Model file for the job. Use its own axes, mm. A direction names the side the tool comes from. Coordinates: 2 decimals unless noted, no trailing zeros. Order: outer loops, then holes, each group sorted by start corner. A loop starts at its lowest first (then second) coordinate and runs counter-clockwise, first axis right, second up. Notation, with made-up numbers: (75, 49) - (89, 49) arc R29 cw to (89, 77) - close; hole circle Ø8 at (66.5, 52.25). An arc over 180 degrees is marked (long way). Put each result on its own line as item: value. Start each with the question number.
```python
from build123d import *

# Parameters (mm, degrees)
SKETCH1_R           = 9.4615
BOSS_EXTRUDE1_DEPTH = 13.97
SKETCH2_R           = 1.905
CUT_EXTRUDE1_DEPTH  = 20.344272137
BOSS_EXTRUDE2_START = 15.24
SKETCH4_R           = 1.905
BOSS_EXTRUDE2_DEPTH = 15.24
FILLET1_R           = 25.4
SKETCH5_R           = 2.286
CUT_EXTRUDE2_DEPTH  = 33.12886653
SKETCH6_R           = 19.05
SKETCH6_R_2         = 9.4615
BOSS_EXTRUDE3_DEPTH = 2.54
SKETCH7_W           = 2.54
SKETCH7_H           = 7.62
CUT_EXTRUDE3_DEPTH  = 40.736999132
CIRPATTERN1_COUNT   = 2


with BuildPart() as part:
    # Sketch1 → Boss-Extrude1 (new body)
    with BuildSketch(Plane(origin=(0, 0, 0), x_dir=(1, 0, 0), z_dir=(0, 1, 0))):
        with Locations(Location((0, 0, 0), (0, 0, 270))):
            Circle(SKETCH1_R)
    extrude(amount=BOSS_EXTRUDE1_DEPTH)

    # Sketch2 → Cut-Extrude1 (cut, through all)
    with BuildSketch(Plane(origin=(0, 13.97, 0), x_dir=(1, 0, 0), z_dir=(0, 1, 0))):
        with Locations(Location((-4.064, 0, 0), (0, 0, 270))):
            Circle(SKETCH2_R)
        with Locations(Location((4.064, 0, 0), (0, 0, 270))):
            Circle(SKETCH2_R)
    extrude(amount=-CUT_EXTRUDE1_DEPTH, mode=Mode.SUBTRACT)

    # Sketch4 → Boss-Extrude2 (add)
    # profile 1 of 2: a face of its own
    with BuildSketch(Plane(origin=(0, 13.97, 0), x_dir=(1, 0, 0), z_dir=(0, 1, 0)).offset(BOSS_EXTRUDE2_START)):
        with BuildLine():
            Line((-0.254, -3.164823692), (-0.254, 3.164823692))
            ThreePointArc((-0.254, 3.164823692), (-0.888489589, 3.048148824), (-1.486296875, 2.805627666))
            ThreePointArc((-1.486296875, 2.805627666), (-7.874, 0), (-1.486296875, -2.805627666))
            ThreePointArc((-1.486296875, -2.805627666), (-0.888489589, -3.048148824), (-0.254, -3.164823692))
        make_face()
        with Locations(Location((-4.064, 0, 0), (0, 0, 270))):
            Circle(SKETCH4_R, mode=Mode.SUBTRACT)
    # profile 2 of 2: a face of its own
    with BuildSketch(Plane(origin=(0, 13.97, 0), x_dir=(1, 0, 0), z_dir=(0, 1, 0)).offset(BOSS_EXTRUDE2_START)):
        with BuildLine():
            ThreePointArc((1.486296875, 2.805627666), (0.888489589, 3.048148824), (0.254, 3.164823692))
            Line((0.254, 3.164823692), (0.254, -3.164823692))
            ThreePointArc((0.254, -3.164823692), (0.888489589, -3.048148824), (1.486296875, -2.805627666))
            ThreePointArc((1.486296875, -2.805627666), (7.874, 0), (1.486296875, 2.805627666))
        make_face()
        with Locations(Location((4.064, 0, 0), (0, 0, 270))):
            Circle(SKETCH4_R, mode=Mode.SUBTRACT)
    extrude(amount=-BOSS_EXTRUDE2_DEPTH)

    # Fillet1
    # the kernel refuses this fillet: 25.4 mm, written as the material it adds along each edge
    with BuildSketch(Plane(origin=(1.486296875, 29.21, -2.805627666), x_dir=(-0.9600468735563171, 0, -0.27983924059134535), z_dir=(0, -1, 0)), Plane(origin=(-1.486296875, 29.21, 2.805627666), x_dir=(0.960046873556317, 0, 0.27983924059134513), z_dir=(0, -1, 0))) as fillet1_piece_1:
        with BuildLine():
            CenterArc((11.360363176, 23.315626496), FILLET1_R, 239.965558217, 6.660918352)
            Line((-1.352857448, 1.32621947), (-1.60712186, 0.886431329))
            ThreePointArc((-1.60712186, 0.886431329), (-0.948303715, 0.385773959), (-0.434645406, -0.262958878))
            Line((-0.434645406, -0.262958878), (0.102686392, -0.497513321))
            ThreePointArc((0.102686392, -0.497513321), (0.641789953, -0.442458258), (1.08204424, -0.46631253))
            Line((1.08204424, -0.46631253), (1.283579905, 0))
        make_face()
    extrude(amount=19.97621774)
    with BuildSketch(Plane(origin=(-1.486296875, 29.21, -2.805627666), x_dir=(-0.881470671461199, 0, -0.4722387694310403), z_dir=(0, -1, 0)), Plane(origin=(1.486296875, 29.21, 2.805627666), x_dir=(0.8814706714611991, 0, 0.47223876943104), z_dir=(0, -1, 0))) as fillet1_piece_2:
        with BuildLine():
            CenterArc((8.209444083, 24.602465695), FILLET1_R, 248.943194802, 6.660918352)
            Line((-0.916607265, 0.898559122), (-1.099128292, 0.424480991))
            ThreePointArc((-1.099128292, 0.424480991), (-0.768042747, 0.133319135), (-0.421608522, -0.283390639))
            Line((-0.421608522, -0.283390639), (0.12629914, -0.492049314))
            ThreePointArc((0.12629914, -0.492049314), (0.947243548, -0.388369854), (1.768187956, -0.492049314))
            Line((1.768187956, -0.492049314), (1.894487096, 0))
        make_face()
    extrude(amount=19.97621774)

    # Sketch5 → Cut-Extrude2 (cut, through all)
    with BuildSketch(Plane.XZ):
        with Locations(Location((0, 6.985, 0), (0, 0, 270))):
            Circle(SKETCH5_R)
        with Locations(Location((0, -6.985, 0), (0, 0, 90))):
            Circle(SKETCH5_R)
    extrude(amount=-CUT_EXTRUDE2_DEPTH, mode=Mode.SUBTRACT)

    # Sketch6 → Boss-Extrude3 (add)
    with BuildSketch(Plane.XZ):
        with Locations(Location((0, 0, 0), (0, 0, 270))):
            Circle(SKETCH6_R)
        with Locations(Location((0, 0, 0), (0, 0, 90))):
            Circle(SKETCH6_R_2, mode=Mode.SUBTRACT)
    extrude(amount=-BOSS_EXTRUDE3_DEPTH)

    # Sketch7 → Cut-Extrude3 (cut, through all)
    with BuildSketch(Plane.XZ):
        with Locations((13.554224028, -1.490382181)):
            Rectangle(SKETCH7_W, SKETCH7_H)
        Polygon((17.364224028, 2.319617819), (14.824224028, 2.319617819), (12.284224028, 2.319617819), (9.744224028, 2.319617819), (13.554224028, 7.399617819), align=None)
    cut_extrude3 = extrude(amount=-CUT_EXTRUDE3_DEPTH, mode=Mode.SUBTRACT)

    # CirPattern1: Cut-Extrude3 ×2 about axis
    cirpattern1_axis = Axis((0, 0, 0), (0, 1, 0))
    for i in range(1, CIRPATTERN1_COUNT):
        add(cut_extrude3.rotate(cirpattern1_axis, i * 360 / CIRPATTERN1_COUNT), mode=Mode.SUBTRACT)


solid = part.part
```
Item 1: 3-axis set-ups, long thin cutter, end or side, ignore diameter. For faces 1 (the face through (-0.254, 22, 0)), 2 (the face through (-15.43, 1.25, -4.9)), 3 (the face through (1.693, 21.697, 3.387)): which of +Z, -Z, +X, -X, +Y, -Y reach the whole face in a straight line?
Item 2: Slice it at B-B, the plane z = 0. Give the number of separate pieces and of enclosed holes in the cut face, plus the area to 3 significant figures.
Item 3: Slice it at C-C, the plane x = -7. Give the cut face in (y, z), plus the area to 3 significant figures.
Item 4: Wall check: line 1 along X through (y, z) = (23.25, 0); line 2 along X through (y, z) = (7, 0); line 3 along X through (y, z) = (11, -1). Give the ranges that are in metal, low to high.
Item 5: Flat gauge pins, fed straight in: pin 1 Ø3 at (y, z) = (21, 1) entering from +X; pin 2 Ø0.8 at (x, y) = (16, 1.5) entering from +Z; pin 3 Ø3 at (y, z) = (11, -10) entering from -X; pin 4 Ø3 at (x, y) = (-9.5, 26) entering from -Z. Where does each tip first touch, or does it go through?
Item 6: Pull direction Z, two halves, no side cores. Call faces 4 (the face through (0, 0, 0)), 5 (the face through (-11.59, 1.25, 15.12)), 6 (the face through (11, 1, 2.32)): pulls with the +Z half, pulls with the -Z half, needs draft (parallel to the pull), parting line crosses it, or undercut.
Item 7: Slice it at D-D, the plane z = 6.5. Give the cut face in (x, y).
Item 8: Slice it at A-A, the plane y = 20.25. Give the cut face in (x, z) (3 decimals).
Here are the results:
1. face 1: +Z, -Z, +Y
1. face 2: +Y, -Y
1. face 3: +Z, +Y
2. separate pieces: 5
2. enclosed holes: 0
2. area: 310 mm^2
3. outline: (0, -17.72) - (2.54, -17.72) - (2.54, -6.37) - (13.97, -6.37) - (13.97, -2.43) - (29.21, -2.43) - (29.21, 2.43) - (13.97, 2.43) - (13.97, 6.37) - (2.54, 6.37) - (2.54, 17.72) - (0, 17.72) - close
3. area: 310 mm^2
4. line 1: x = -7.87 to -5.97, -2.16 to -0.25, 0.25 to 2.16, 5.97 to 7.87
4. line 2: x = -9.46 to -5.97, -2.16 to 2.16, 5.97 to 9.46
4. line 3: x = -9.41 to -5.69, -2.44 to 2.44, 5.69 to 9.41
5. pin 1: stops at x = 7.87
5. pin 2: stops at z = 10.93
5. pin 3: stops at x = -4.16
5. pin 4: passes through
6. face 4: needs draft
6. face 5: parting line crosses it
6. face 6: undercut
7. outline: (-17.91, 0) - (-2.23, 0) - (-2.23, 13.97) - (-6.88, 13.97) - (-6.88, 2.54) - (-17.91, 2.54) - close; (2.23, 0) - (12.88, 0) - (12.88, 2.54) - (6.88, 2.54) - (6.88, 13.97) - (2.23, 13.97) - close; (14.23, 0) - (17.91, 0) - (17.91, 2.54) - (14.23, 2.54) - close
8. outline: (-3.156, -3.7) arc R25.4 cw to (-0.254, -3.165) - (-0.254, 3.165) arc R25.4 cw to (-3.156, 3.7) arc R3.81 ccw (long way) to start; (0.254, -3.165) arc R25.4 cw to (3.156, -3.7) arc R3.81 ccw (long way) to (3.156, 3.7) arc R25.4 cw to (0.254, 3.165) - close; hole circle Ø3.81 at (-4.064, 0); hole circle Ø3.81 at (4.064, 0)
